Here's how the part is built. I have some questions about the finished solid (model axes, mm). Face numbers are marked on the shaded views. Round coordinates to 2 decimals unless told otherwise and drop trailing zeros. Write each loop counter-clockwise with the first axis right and the second up, starting at its lowest first coordinate (ties: lowest second). Pieces come first, ordered by that corner, then holes. Notation, with made-up numbers: (54, 40.5) -> (89, 40.5) arc R28 ccw to (89, 72.5) -> close; hole circle Ø10 at (-4, 40). An arc over 180 degrees is marked (long way). Answer in a Markdown table with one row per item.
from build123d import *

# Parameters (mm, degrees)
SKETCH1_R               = 6.35
SKETCH1_R_2             = 2.5527
BOSS_EXTRUDE1_DEPTH     = 31.75
SKETCH2_R               = 12.7
SKETCH2_R_2             = 2.5527
BOSS_EXTRUDE2_DEPTH     = 6.35
SKETCH3_R               = 0.5953125
CUT_EXTRUDE1_DEPTH      = 43.121134838
BOSS_EXTRUDE3_START     = -38.1
SKETCH11_R              = 2.5527
BOSS_EXTRUDE3_DEPTH     = 38.1
F_1_4_20_TAPPED_HOLE3_D = 5.1054


with BuildPart() as part:
    # Sketch1 → Boss-Extrude1 (new body)
    with BuildSketch(Plane.XY):
        Circle(SKETCH1_R)
        Circle(SKETCH1_R_2, mode=Mode.SUBTRACT)
    extrude(amount=BOSS_EXTRUDE1_DEPTH)

    # Sketch2 → Boss-Extrude2 (add)
    with BuildSketch(Plane.XY.offset(31.75)):
        Circle(SKETCH2_R)
        Circle(SKETCH2_R_2, mode=Mode.SUBTRACT)
    extrude(amount=BOSS_EXTRUDE2_DEPTH)

    # Sketch3 → Cut-Extrude1 (cut, through all)
    with BuildSketch(Plane.XY.offset(38.1)):
        with Locations((-7.62, 0)):
            Circle(SKETCH3_R)
        with Locations((7.62, 0)):
            Circle(SKETCH3_R)
    extrude(amount=-CUT_EXTRUDE1_DEPTH, mode=Mode.SUBTRACT)

    # Sketch11 → Boss-Extrude3 (add)
    with BuildSketch(Plane.XY.offset(38.1).offset(BOSS_EXTRUDE3_START)):
        Circle(SKETCH11_R)
    extrude(amount=BOSS_EXTRUDE3_DEPTH)

    # 1/4-20 Tapped Hole3 (through all)
    with Locations(Plane.XY.offset(38.1)):
        with Locations((0, 0)):
            Hole(F_1_4_20_TAPPED_HOLE3_D / 2)


solid = part.part
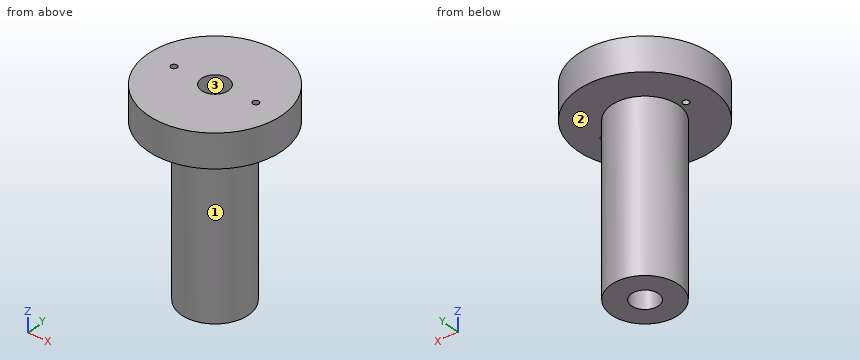
1) I want a section at A-A, the plane x = 7.62. List the corners of the cut face in (y, z) for me.
Response:
| item | result |
|---|---|
| outline | (-10.16, 31.75) -> (-0.6, 31.75) -> (-0.6, 38.1) -> (-10.16, 38.1) -> close; (0.6, 31.75) -> (10.16, 31.75) -> (10.16, 38.1) -> (0.6, 38.1) -> close |
2) I want a section at C-C, the plane z = 22.5. List the corners of the cut face in (x, y) for me, and give its area (3 significant figures).
Response:
| item | result |
|---|---|
| outline | circle Ø12.7 at (0, 0); hole circle Ø5.11 at (0, 0) |
| area | 106 mm^2 |
3) I want a section at D-D, the plane y = 4. List the corners of the cut face in (x, z) for me, and give its area (3 significant figures).
Response:
| item | result |
|---|---|
| outline | (-12.05, 31.75) -> (-4.93, 31.75) -> (-4.93, 0) -> (4.93, 0) -> (4.93, 31.75) -> (12.05, 31.75) -> (12.05, 38.1) -> (-12.05, 38.1) -> close |
| area | 466 mm^2 |
4) I need wall thicknesses on line 1 (Z direction, x = -5.5, y = 5.5); line 2 (Y direction, x = -7.62, z = 34); line 3 (X direction, y = 0.25, z = 9.5). Which ranges of each line are inside material? Lowest first, please. Write a range as [from, to].
Response:
| item | result |
|---|---|
| line 1 | z = [31.75, 38.1] |
| line 2 | y = [-10.16, -0.6], [0.6, 10.16] |
| line 3 | x = [-6.35, -2.54], [2.54, 6.35] |
5) We'd pull the mould along X, two halves only. Please class the marked faces 1, 2 and 3: +X half, -X half, draft (parallel to the pull), parting line (faces both ways), or undercut.
Response:
| item | result |
|---|---|
| face 1 | parting line |
| face 2 | draft |
| face 3 | undercut |
6) I want a section at B-B, the plane y = 0. List the corners of the cut face in (x, z) for me, and give its area (3 significant figures).
Response:
| item | result |
|---|---|
| outline | (-12.7, 31.75) -> (-8.22, 31.75) -> (-8.22, 38.1) -> (-12.7, 38.1) -> close; (-7.02, 31.75) -> (-6.35, 31.75) -> (-6.35, 0) -> (-2.55, 0) -> (-2.55, 38.1) -> (-7.02, 38.1) -> close; (2.55, 0) -> (6.35, 0) -> (6.35, 31.75) -> (7.02, 31.75) -> (7.02, 38.1) -> (2.55, 38.1) -> close; (8.22, 31.75) -> (12.7, 31.75) -> (12.7, 38.1) -> (8.22, 38.1) -> close |
| area | 355 mm^2 |
7) For pin 1 (3 mm diameter, centred on x = 8, y = -5, fed in from -Z); pin 2 (12 mm diameter, centred on x = -4.5, z = 16.5, fed in from +Y); pin 3 (1.4 mm diameter, centred on x = 7.62, y = 0, fed in from +Z); pin 4 (8 mm diameter, centred on x = 8, z = 23, fed in from -Y), each with a flat end and sliding along its axis, tell me the tip position at first contact or that it passes through.
Response:
| item | result |
|---|---|
| pin 1 | stops at z = 31.75 |
| pin 2 | stops at y = 6.35 |
| pin 3 | stops at z = 38.1 |
| pin 4 | stops at y = -4.93 |
